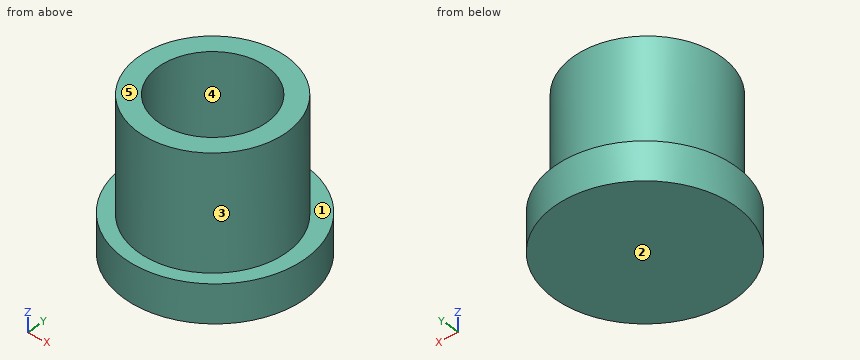
```python
from build123d import *

# Parameters (mm, degrees)
F0_R     = 83.5800069383
F0_R_2   = 61.6002639071
F1_DEPTH = 381
F2_DEPTH = 127
F4_R     = 48.4229343949
F4_R_2   = 35.527059512
F5_DEPTH = 100
F6_R     = 59.1924644961
F7_DEPTH = 25


with BuildPart() as f1:
    # F0 (on Top) → F1 (new body)
    with BuildSketch(Plane.XY):
        with Locations((-408.8018536568, 0)):
            Circle(F0_R)
        with Locations((-408.8018536568, 0)):
            Circle(F0_R_2, mode=Mode.SUBTRACT)
    extrude(amount=F1_DEPTH)

    # F2 (add): a face of the model
    f2_faces = [f1.faces().sort_by_distance(p)[0] for p in [
        (-490.0178610079, 0, 381),
    ]]
    extrude(f2_faces, amount=F2_DEPTH)


with BuildPart() as f5:
    # F4 (on Top) → F5 (new body)
    with BuildSketch(Plane.XY):
        with Locations((-174.1937100887, 12.2994268313)):
            Circle(F4_R)
        with Locations((-174.1937100887, 12.2994268313)):
            Circle(F4_R_2, mode=Mode.SUBTRACT)
    extrude(amount=F5_DEPTH)

    # F6 (on Top) → F7 (join)
    with BuildSketch(Plane.XY):
        with Locations((-174.5279580355, 14.4501468167)):
            Circle(F6_R)
    extrude(amount=F7_DEPTH)


solid = f5.part
```
The model under review builds one solid part; all positions refer to its coordinate system, in mm. Face numbers are marked on the shaded views. A direction names the side the tool comes from. Coordinates: 2 decimals unless noted, no trailing zeros. Order: outer loops, then holes, each group sorted by start corner. A loop starts at its lowest first (then second) coordinate and runs counter-clockwise, first axis right, second up. Notation, with made-up numbers: M -9.5,49.5 L 15.5,49.5 A20 ccw 15.5,69.5 Z; hole C -5.75,-35.5 d7. An arc over 180 degrees is marked long. One line per question, with ' | ' between items.
(1) Add section A-A, the plane y = -28.5. Write out the cut boundary in (x, z), then the cut area to 3 significant figures.
Geometry results:
outline: M -215.26,0 L -133.8,0 L -133.8,25 L -148.11,25 L -148.11,100 L -200.27,100 L -200.27,25 L -215.26,25 Z | area: 5,950 mm²
(2) Add section D-D, the plane y = 44.5. Write out the cut boundary in (x, z), then the cut area to 3 significant figures.
Geometry results:
outline: M -225.53,0 L -123.53,0 L -123.53,25 L -138.03,25 L -138.03,100 L -159.18,100 L -159.18,25 L -189.2,25 L -189.2,100 L -210.36,100 L -210.36,25 L -225.53,25 Z | area: 5,720 mm²
(3) For probe 1 along Z at (x, y) = (-173.5, 12.5); probe 2 along Y at (x, z) = (-206, 82); probe 3 along Y at (x, z) = (-150.5, 58.5), list the stretches that pass through material, from the lowest coordinate up. Write a range as from..to.
Geometry results:
probe 1: z = 0..25 | probe 2: y = -24.21..-3.53, 28.13..48.81 | probe 3: y = -29.93..-14.17, 38.77..54.53
(4) Machinability: for the marked faces 1 and 2, which of the approach directions +Z, -Z, +X, -X, +Y, -Y give a long, thin tool a straight path to every point of the face, cutting with its end or side? Answer none if there is none.
Geometry results:
face 1: +Z | face 2: -Z, +X, -X, +Y, -Y
(5) Insertion check: pin 1 (8 mm diameter, centred on x = -163.5, z = 36, fed in from +Y); pin 2 (8 mm diameter, centred on y = 36, z = 82.5, fed in from -X); pin 3 (1 mm diameter, centred on x = -180, z = 68.5, fed in from +Y). Each pin has a flat end and moves straight along its axis. Give the tip position at first contact, or say it passes through.
Geometry results:
pin 1: stops at y = 60.26 | pin 2: stops at x = -218.43 | pin 3: stops at y = 60.43
(6) The part is to be moulded in two halves that separate along Y. For the marked faces 3, 4 and 5, say which applies: +Y half, -Y half, draft (parallel to the pull), parting line (faces both ways), or undercut.
Geometry results:
face 3: parting line | face 4: undercut | face 5: draft
(7) Add section B-B, the plane x = -192.5. Write out the cut boundary in (y, z), then the cut area to 3 significant figures.
Geometry results:
outline: M -41.95,0 L 70.85,0 L 70.85,25 L 57.13,25 L 57.13,100 L 42.75,100 L 42.75,25 L -18.15,25 L -18.15,100 L -32.53,100 L -32.53,25 L -41.95,25 Z | area: 4,980 mm²
(8) Add section C-C, the plane z = 59.5. Write out the cut boundary in (x, y), then the cut area to 3 significant figures.
Geometry results:
outline: C -174.19,12.3 d96.85; hole C -174.19,12.3 d71.05 | area: 3,400 mm²
